from build123d import *

# Parameters (mm, degrees)
F0_W     = 50.8
F0_H     = 76.2
F1_DEPTH = 25.4
F2_R     = 5.08
F3_R     = 12.7
F4_DEPTH = 50.801
F5_R     = 9.300701
F6_DEPTH = 76.201


with BuildPart() as f1:
    # F0 (on Top) → F1 (new body, symmetric)
    with BuildSketch(Plane.XY):
        Rectangle(F0_W, F0_H)
    extrude(amount=F1_DEPTH, both=True)

    # F2
    f2_edges = [f1.edges().sort_by_distance(p)[0] for p in [
        (25.4, 0, 25.4),
        (25.4, -38.1, 0),
        (0, -38.1, 25.4),
    ]]
    fillet(f2_edges, radius=F2_R)

    # F3 (on face) → F4 (cut, through all)
    with BuildSketch(Plane.YZ.offset(25.4)):
        Circle(F3_R)
    extrude(amount=-F4_DEPTH, mode=Mode.SUBTRACT)

    # F5 (on face) → F6 (cut, through all)
    with BuildSketch(Plane.XZ.offset(38.1)):
        with Locations((-14.431597, 4.293228)):
            Circle(F5_R)
    extrude(amount=-F6_DEPTH, mode=Mode.SUBTRACT)


solid = f1.part
Input: part model. Units: mm. Frame: model coordinates. Round coordinates to 2 decimals unless told otherwise and drop trailing zeros. Order: outer loops, then holes, each group sorted by start corner. A loop starts at its lowest first (then second) coordinate and runs counter-clockwise, first axis right, second up.
1. Mould query, pull axis Z, two halves, no side actions, for faces 1 (the face through (6, -2.75, -12.4)), 2 (the face through (-15.642, -0.533, 13.515)), 3 (the face through (23.872, 3.038, 23.951)), 4 (the face through (23.951, -36.572, -2.22)). Classes: released by +Z, released by -Z, zero draft, split by the parting line, or undercut.
The answers:
face 1: undercut
face 2: undercut
face 3: released by +Z
face 4: zero draft
2. Cut plane A-A, the plane y = 3.5. Output: boundary loops of the cut face in (x, z).
The answers:
outline: (-25.4, -25.4) - (25.4, -25.4) - (25.4, -12.21) - (-25.4, -12.21) - close; (-25.4, 12.21) - (-19.32, 12.21) arc R9.3 cw to (-9.55, 12.21) - (25.4, 12.21) - (25.4, 20.32) arc R5.08 ccw to (20.32, 25.4) - (-25.4, 25.4) - close
3. Cut plane B-B, the plane x = -17. Output: boundary loops of the cut face in (y, z).
The answers:
outline: (-38.1, -25.4) - (38.1, -25.4) - (38.1, -4.65) - (11.82, -4.65) arc R12.7 cw to (-11.82, -4.65) - (-38.1, -4.65) - close; (-38.1, 13.23) - (38.1, 13.23) - (38.1, 25.4) - (-33.02, 25.4) arc R5.08 ccw to (-38.1, 20.32) - close
4. Cut plane D-D, the plane x = 15.5. Output: boundary loops of the cut face in (y, z), then the cut area to 3 significant figures.
The answers:
outline: (-38.1, -25.4) - (38.1, -25.4) - (38.1, 25.4) - (-33.02, 25.4) arc R5.08 ccw to (-38.1, 20.32) - close; hole circle Ø25.4 at (0, 0)
area: 3,360 mm2
5. Cut plane C-C, the plane z = 0. Output: boundary loops of the cut face in (x, y).
The answers:
outline: (-25.4, -38.1) - (-22.68, -38.1) - (-22.68, -12.7) - (-25.4, -12.7) - close; (-25.4, 12.7) - (-22.68, 12.7) - (-22.68, 38.1) - (-25.4, 38.1) - close; (-6.18, -38.1) - (20.32, -38.1) arc R5.08 ccw to (25.4, -33.02) - (25.4, -12.7) - (-6.18, -12.7) - close; (-6.18, 12.7) - (25.4, 12.7) - (25.4, 38.1) - (-6.18, 38.1) - close
6. Material intervals for line 1 (Z direction, x = -15, y = -32); line 2 (Y direction, x = 14, z = 0); line 3 (Z direction, x = 0.5, y = 0), sorted ascending.
The answers:
line 1: z = -25.4 to -4.99, 13.58 to 25.4
line 2: y = -38.1 to -12.7, 12.7 to 38.1
line 3: z = -25.4 to -12.7, 12.7 to 25.4
7. Pin query (flat end, axial travel): P1, Ø16.5, axis at x = -14.43, z = 4.29, coming from the -Y side. Return the tip coordinate at first contact, or that it passes through.
The answers:
P1: passes through
